CAD build for the part. Positions are in the model's coordinates, mm. Face numbers are marked on the shaded views. Coordinates: 2 decimals unless noted, no trailing zeros. Loops run counter-clockwise (first coordinate to the right, second up) from the corner with the lowest first, then second, coordinate; pieces in that order, holes last. Notation, with made-up numbers: (-1, 86.5) -> (11, 86.5) arc R29 ccw to (11, 107.5) -> close; hole circle Ø2 at (8.25, 52). An arc over 180 degrees is marked (long way). Write each question's results on one line, items separated by ' | '.
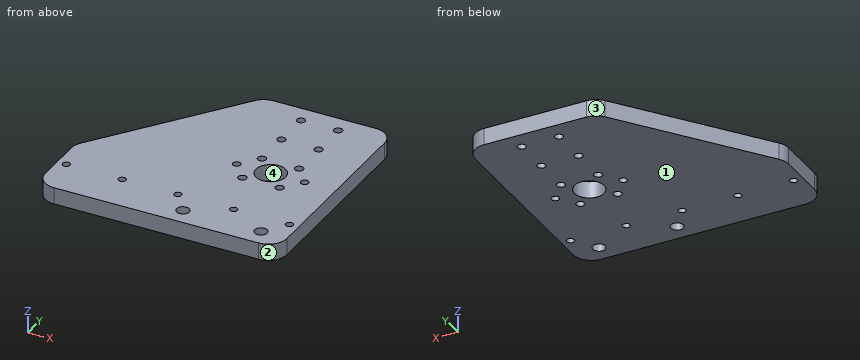
```python
from build123d import *

# Parameters (mm, degrees)
BOSS_EXTRU_1_DEPTH      = 9
ESQUISSE2_R             = 2
ESQUISSE2_R_2           = 2.25
ENL_V_MAT_EXTRU_1_DEPTH = 178.146831753
ESQUISSE3_R             = 8
ESQUISSE3_R_2           = 3.4
ENL_V_MAT_EXTRU_2_DEPTH = 178.146831753
CONG_1_R                = 10
ESQUISSE6_R             = 2.1
ENL_V_MAT_EXTRU_4_DEPTH = 178.146831753


with BuildPart() as part:
    # Esquisse1 → Boss.-Extru.1 (new body)
    with BuildSketch(Plane.XY):
        Polygon((0, 0), (130, 0), (130, 120), (60, 120), (0, 40), align=None)
    extrude(amount=BOSS_EXTRU_1_DEPTH)

    # Esquisse2 → Enlèv. mat.-Extru.1 (cut, through all)
    with BuildSketch(Plane.XY.offset(9)):
        with Locations((65, 22)):
            Circle(ESQUISSE2_R)
        with Locations((35, 22)):
            Circle(ESQUISSE2_R)
        with Locations((5, 22)):
            Circle(ESQUISSE2_R)
        with Locations(Location((125, 22, 0), (0, 0, 180))):
            Circle(ESQUISSE2_R)
        with Locations(Location((95, 22, 0), (0, 0, 180))):
            Circle(ESQUISSE2_R)
        with Locations((85, 110)):
            Circle(ESQUISSE2_R_2)
        with Locations(Location((85, 90, 0), (0, 0, 180))):
            Circle(ESQUISSE2_R_2)
        with Locations((105, 90)):
            Circle(ESQUISSE2_R_2)
        with Locations(Location((105, 110, 0), (0, 0, 180))):
            Circle(ESQUISSE2_R_2)
        with Locations((105, 50)):
            Circle(ESQUISSE2_R_2)
        with Locations(Location((105, 70, 0), (0, 0, 180))):
            Circle(ESQUISSE2_R_2)
        with Locations((85, 70)):
            Circle(ESQUISSE2_R_2)
        with Locations(Location((85, 50, 0), (0, 0, 180))):
            Circle(ESQUISSE2_R_2)
    extrude(amount=-ENL_V_MAT_EXTRU_1_DEPTH, mode=Mode.SUBTRACT)

    # Esquisse3 → Enlèv. mat.-Extru.2 (cut, through all)
    with BuildSketch(Plane.XY.offset(9)):
        with Locations((95, 60)):
            Circle(ESQUISSE3_R)
        with Locations((74, 10)):
            Circle(ESQUISSE3_R_2)
        with Locations(Location((116, 10, 0), (0, 0, 180))):
            Circle(ESQUISSE3_R_2)
    extrude(amount=-ENL_V_MAT_EXTRU_2_DEPTH, mode=Mode.SUBTRACT)

    # Congé1
    cong_1_edges = [part.edges().sort_by_distance(p)[0] for p in [
        (0, 40, 4.5),
        (60, 120, 4.5),
        (130, 120, 4.5),
        (130, 0, 4.5),
        (0, 0, 4.5),
    ]]
    fillet(cong_1_edges, radius=CONG_1_R)

    # Esquisse6 → Enlèv. mat.-Extru.4 (cut, through all)
    with BuildSketch(Plane(origin=(0, 0, 0), x_dir=(-1, 0, 0), z_dir=(0, 0, -1))):
        with Locations((-113.25, 60)):
            Circle(ESQUISSE6_R)
        with Locations(Location((-76.75, 60, 0), (0, 0, 180))):
            Circle(ESQUISSE6_R)
    extrude(amount=-ENL_V_MAT_EXTRU_4_DEPTH, mode=Mode.SUBTRACT)


solid = part.part
```
Q1. Cut at A-A on y = 60. Write the cut outline in (x, z).
Results are:
outline: (15, 0) -> (74.65, 0) -> (74.65, 9) -> (15, 9) -> close; (78.85, 0) -> (87, 0) -> (87, 9) -> (78.85, 9) -> close; (103, 0) -> (111.15, 0) -> (111.15, 9) -> (103, 9) -> close; (115.35, 0) -> (130, 0) -> (130, 9) -> (115.35, 9) -> close
Q2. Cut at B-B on x = 85. Write the cut outline in (y, z).
Results are:
outline: (0, 0) -> (47.75, 0) -> (47.75, 9) -> (0, 9) -> close; (52.25, 0) -> (67.75, 0) -> (67.75, 9) -> (52.25, 9) -> close; (72.25, 0) -> (87.75, 0) -> (87.75, 9) -> (72.25, 9) -> close; (92.25, 0) -> (107.75, 0) -> (107.75, 9) -> (92.25, 9) -> close; (112.25, 0) -> (120, 0) -> (120, 9) -> (112.25, 9) -> close
Q3. Pull direction X, two halves, no side cores. Call the marked faces 1, 2, 3 and 4: +X half, -X half, draft (parallel to the pull), parting line (faces both ways), or undercut.
Results are:
face 1: draft | face 2: +X half | face 3: -X half | face 4: undercut
Q4. Cut at C-C on z = 1.5. Give the number of separate pieces and of enclosed holes in the cut face, and give its area (3 significant figures).
Results are:
separate pieces: 1 | enclosed holes: 18 | area: 12,600 mm^2
Q5. Cut at D-D on y = 22. Write the cut outline in (x, z), and give its area (3 significant figures).
Results are:
outline: (0, 0) -> (3, 0) -> (3, 9) -> (0, 9) -> close; (7, 0) -> (33, 0) -> (33, 9) -> (7, 9) -> close; (37, 0) -> (63, 0) -> (63, 9) -> (37, 9) -> close; (67, 0) -> (93, 0) -> (93, 9) -> (67, 9) -> close; (97, 0) -> (123, 0) -> (123, 9) -> (97, 9) -> close; (127, 0) -> (130, 0) -> (130, 9) -> (127, 9) -> close | area: 990 mm^2
Q6. Wall check: L1, parallel to Y at x = 105, z = 5.25; L2, parallel to Y at x = 95, z = 5; L3, parallel to Y at x = 113.25, z = 5.75. Give the ranges that are in metal, low to high. Write a range as from..to.
Results are:
L1: 0..47.75, 52.25..67.75, 72.25..87.75, 92.25..107.75, 112.25..120 | L2: 0..20, 24..52, 68..120 | L3: 0..8, 12..57.9, 62.1..120
Q7. Drop flat-ended pins along their axis: pin 1 (6 mm diameter, centred on x = 74, y = 10, fed in from -Z); pin 2 (2 mm diameter, centred on y = 78, z = 4.5, fed in from -X). Give the stop position or say it passes through.
Results are:
pin 1: through | pin 2: x = 27.75
